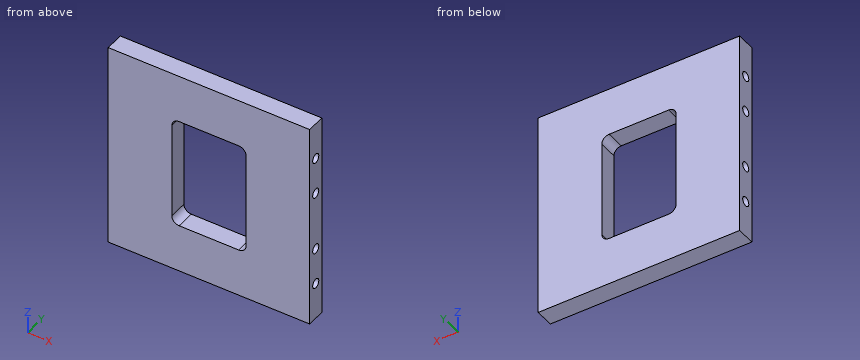
Autodesk Inventor part; units mm, degrees
ref_plane "YZ Plane" through (0, 0, 0) normal (1, 0, 0) x (0, 1, 0)
ref_plane "XZ Plane" through (0, 0, 0) normal (0, 1, 0) x (-1, 0, 0)
ref_plane "XY Plane" through (0, 0, 0) normal (0, 0, 1) x (1, 0, 0)
sketch "스케치1" plane through (0, 0, 0) normal (0, 1, 0) x (-1, 0, 0)
  line L0 (27.1, 28) -> (-27.1, 28)
  line L1 (-27.1, 28) -> (-27.1, -28)
  line L2 (-27.1, -28) -> (27.1, -28)
  line L3 (27.1, -28) -> (27.1, 28)
  point P0 (0, 0)
  dimension "d0" = 54.2
  dimension "d1" = 56
  dimension "d2" = 27.1
  dimension "d3" = 28
extrude "돌출1" add sketch "스케치1" along normal blind 5
sketch "스케치5" plane through (27.1, 0, 28) normal (1, 0, 0) x (0, 0, -1)
  line L0 (0, 0) -> (56, 0)
  line L1 (56, 0) -> (56, 5)
  line L2 (0, 5) -> (56, 5)
  line L3 (0, 0) -> (0, 5)
  circle A0 centre (10, 2.5) radius 1.25
  circle A1 centre (20, 2.5) radius 1.25
  circle A2 centre (46, 2.5) radius 1.25
  circle A3 centre (36, 2.5) radius 1.25
  point P0 (28, 0)
  dimension "d16" = 2.5
  dimension "d17" = 2.5
  dimension "d18" = 2.5
  dimension "d19" = 2.5
  dimension "d20" = 2.5
  dimension "d21" = 2.5
  dimension "d22" = 2.5
  dimension "d23" = 2.5
  dimension "d24" = 10
  dimension "d25" = 20
  dimension "d26" = 20
  dimension "d27" = 10
extrude "돌출5" cut sketch "스케치5" against normal blind 8 contours A0 | A1 | A2 | A3
sketch "스케치6" plane through (-27.1, 0, -28) normal (-1, 0, 0) x (0, 0, 1)
  circle A0 centre (10, 2.5) radius 1.25
  circle A1 centre (46, 2.5) radius 1.25
  circle A2 centre (36, 2.5) radius 1.25
  circle A3 centre (20, 2.5) radius 1.25
  line L0 (56, 0) -> (0, 0)
  line L1 (0, 0) -> (0, 5)
  line L2 (56, 5) -> (0, 5)
  line L3 (56, 0) -> (56, 5)
  point P0 (28, 0)
extrude "돌출6" cut sketch "스케치6" against normal blind 8 contours A0 | A1 | A2 | A3
sketch "스케치7" plane through (0, 5, 0) normal (0, 1, 0) x (1, 0, 0)
  line L0 (-10, 15) -> (10, 15)
  line L1 (10, 15) -> (10, -15)
  line L2 (10, -15) -> (-10, -15)
  line L3 (-10, -15) -> (-10, 15)
  point P0 (0, 0)
  dimension "d32" = 20
  dimension "d33" = 30
  dimension "d34" = 10
  dimension "d35" = 15
extrude "돌출7" cut sketch "스케치7" against normal up to surface (5 mm away)
fillet "모깎기1" radius 2 4 edges at (-10, 2.5, -15) (10, 2.5, -15) (-10, 2.5, 15) (10, 2.5, 15)
properties part number "J1J2_Bottom" material "알루미늄 6061"
Part model, mm, in its own coordinate system. Give positions to 0.01 mm unless a question says otherwise; leave off trailing zeros. Loops run counter-clockwise (first coordinate to the right, second up) from the corner with the lowest first, then second, coordinate; pieces in that order, holes last. Notation, with made-up numbers: (18.5, 34.25) -> (64.5, 34.25) arc R24 ccw to (64.5, 52.25) -> close; hole circle Ø1 at (34, 34). An arc over 180 degrees is marked (long way). Write each question's results on one line, items separated by ' | '. Start each with the question number.
Q1. Band-saw the part on B-B on x = -22. List the corners of the cut face in (y, z), plus the area to 3 significant figures.
Q2. Wall check: L1, parallel to Z at x = -1, y = 1.1; L2, parallel to X at y = 3.5, z = 2; L3, parallel to Y at x = -25, z = -8. Give the ranges that are in metal, low to high.
Q3. Band-saw the part on A-A on z = 8. List the corners of the cut face in (x, y).
Q4. Pin check, flat tips, straight feed: P1, Ø3, axis at y = 2.5, z = 8, coming from the -X side; P2, Ø2, axis at y = 2.5, z = -8, coming from the -X side; P3, Ø1.2, axis at y = 2.5, z = -17.5, coming from the +X side. Stop position of each tip, or through.
Q5. Band-saw the part on C-C on x = -9. List the corners of the cut face in (y, z).
Q6. Band-saw the part on D-D on z = 18. List the corners of the cut face in (x, y), plus the area to 3 significant figures.
Results are:
1) outline: (0, -28) -> (5, -28) -> (5, 28) -> (0, 28) -> close; hole circle Ø2.5 at (2.5, -18); hole circle Ø2.5 at (2.5, -8); hole circle Ø2.5 at (2.5, 8); hole circle Ø2.5 at (2.5, 18) | area: 260 mm²
2) L1: z = -28 to -15, 15 to 28 | L2: x = -27.1 to -10, 10 to 27.1 | L3: y = 0 to 1.25, 3.75 to 5
3) outline: (-27.1, 0) -> (-10, 0) -> (-10, 5) -> (-27.1, 5) -> (-27.1, 3.75) -> (-19.1, 3.75) -> (-19.1, 1.25) -> (-27.1, 1.25) -> close; (10, 0) -> (27.1, 0) -> (27.1, 1.25) -> (19.1, 1.25) -> (19.1, 3.75) -> (27.1, 3.75) -> (27.1, 5) -> (10, 5) -> close
4) P1: stops at x = -27.1 | P2: stops at x = -19.1 | P3: stops at x = 19.1
5) outline: (0, -28) -> (5, -28) -> (5, -14.73) -> (0, -14.73) -> close; (0, 14.73) -> (5, 14.73) -> (5, 28) -> (0, 28) -> close
6) outline: (-27.1, 0) -> (27.1, 0) -> (27.1, 1.25) -> (19.1, 1.25) -> (19.1, 3.75) -> (27.1, 3.75) -> (27.1, 5) -> (-27.1, 5) -> (-27.1, 3.75) -> (-19.1, 3.75) -> (-19.1, 1.25) -> (-27.1, 1.25) -> close | area: 231 mm²
